from build123d import *

# Parameters (mm, degrees)
F1_DEPTH = 6
F2_R     = 0.25
F3_DEPTH = 25
F4_W     = 3
F4_H     = 0.5
F5_DEPTH = 25


with BuildPart() as f1:
    # F0 (on Right) → F1 (new body)
    with BuildSketch(Plane.YZ):
        Polygon((0, 2), (0, 0), (5, 0), (5, 2), (2.875, 2), (2.875, 1.5), (3.5, 1.5), (3.5, 1), (1.5, 1), (1.5, 1.5), (2.125, 1.5), (2.125, 2), align=None)
    extrude(amount=F1_DEPTH)

    # F2 (on face) → F3 (cut)
    with BuildSketch(Plane.XY.offset(2)):
        with Locations((0.75, 0.75)):
            Circle(F2_R)
        with Locations((5.25, 0.75)):
            Circle(F2_R)
    extrude(amount=-F3_DEPTH, mode=Mode.SUBTRACT)

    # F4 (on face) → F5 (cut)
    with BuildSketch(Plane.XZ):
        with Locations((3, 0.25)):
            Rectangle(F4_W, F4_H)
    extrude(amount=-F5_DEPTH, mode=Mode.SUBTRACT)


solid = f1.part
Work out the finished part from the listing and answer in its coordinate system (mm). A direction names the side the tool comes from. Coordinates: 2 decimals unless noted, no trailing zeros. Loops run counter-clockwise (first coordinate to the right, second up) from the corner with the lowest first, then second, coordinate; pieces in that order, holes last. Notation, with made-up numbers: M 11.25,70 L 36.25,70 A14 cw 36.25,85 Z; hole C 28,62.25 d3. An arc over 180 degrees is marked long. Answer in a Markdown table with one row per item. Add a question column.
1. Find section B-B, the plane y = 0.75. Write down the section's boundary in (x, z), then the cut area to 3 significant figures.
2. A tool of negligible diameter and unlimited length cuts with its end or side. For faces 4 (the flat face through (3, 0, 1)), 5 (the flat face through (3, 2, 0.5)), from which of +Z, -Z, +X, -X, +Y, -Y can it reach the whole face along a straight path? Write none if from no direction.
3. Find section A-A, the plane z = 1.15. Write down the section's boundary in (x, y).
4. Find section D-D, the plane y = 1.75. Write down the section's boundary in (x, z).
5. Consider L1, parallel to Y at x = 5.25, z = 1.3; L2, parallel to X at y = 2.55, z = 0.3; L3, parallel to Y at x = 3.2, z = 1.8 (3 decimals). Determine where each line is inside the solid, lowest interval first.
6. The mould has two halves that part along Z. Classify faces 1 (the flat face through (6, 2.5, 0.8)), 2 (the flat face through (3, 3, 1)), 3 (the flat face through (3, 4, 2)): pulls with the +Z half, pulls with the -Z half, needs draft (parallel to the pull), parting line crosses it, or undercut.
7. A flat-ended cylindrical pin translates along its axis: P1, Ø0.7, axis at x = 3.5, y = 1.5, coming from the -Z side. Find the tip coordinate at first contact, or state that the pin passes through.
8. Find section C-C, the plane x = 3.15. Write down the section's boundary in (y, z) (3 decimals), then the cut area to 4 significant figures.
Reported:
| question | item | result |
|---|---|---|
| 1 | outline | M 0,0 L 0.5,0 L 0.5,2 L 0,2 Z; M 1,0 L 1.5,0 L 1.5,0.5 L 4.5,0.5 L 4.5,0 L 5,0 L 5,2 L 1,2 Z; M 5.5,0 L 6,0 L 6,2 L 5.5,2 Z |
| 1 | area | 8.50 mm^2 |
| 2 | face 4 | +Z, -Z, +X, -X, -Y |
| 2 | face 5 | -Z, +Y, -Y |
| 3 | outline | M 0,0 L 6,0 L 6,1.5 L 0,1.5 Z; M 0,3.5 L 6,3.5 L 6,5 L 0,5 Z; hole C 0.75,0.75 d0.5; hole C 5.25,0.75 d0.5 |
| 4 | outline | M 0,0 L 1.5,0 L 1.5,0.5 L 4.5,0.5 L 4.5,0 L 6,0 L 6,1 L 0,1 Z; M 0,1.5 L 6,1.5 L 6,2 L 0,2 Z |
| 5 | L1 | y = 0 to 0.5, 1 to 1.5, 3.5 to 5 |
| 5 | L2 | x = 0 to 1.5, 4.5 to 6 |
| 5 | L3 | y = 0 to 2.125, 2.875 to 5 |
| 6 | face 1 | needs draft |
| 6 | face 2 | undercut |
| 6 | face 3 | pulls with the +Z half |
| 7 | P1 | stops at z = 0.5 |
| 8 | outline | M 0,0.5 L 5,0.5 L 5,2 L 2.875,2 L 2.875,1.5 L 3.5,1.5 L 3.5,1 L 1.5,1 L 1.5,1.5 L 2.125,1.5 L 2.125,2 L 0,2 Z |
| 8 | area | 6.125 mm^2 |
